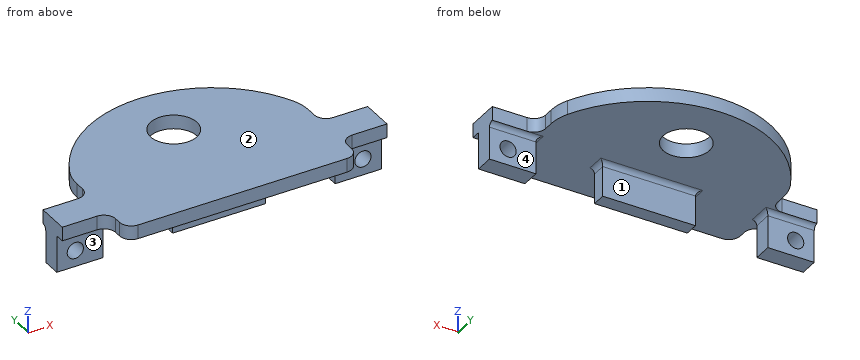
```python
from build123d import *

# Parameters (mm, degrees)
SKETCH1_W           = 20
SKETCH1_H           = 155
BOSS_EXTRUDE1_DEPTH = 4
SKETCH2_W           = 20
SKETCH2_H           = 4
BOSS_EXTRUDE3_DEPTH = 50
RIB2_REACH          = 96.986
SKETCH7_WALL_W      = 290.205463948
SKETCH7_WALL_H      = 4
SKETCH8_W           = 20
SKETCH8_H           = 3
BOSS_EXTRUDE4_DEPTH = 3.5
SKETCH9_W           = 70
SKETCH9_H           = 5
BOSS_EXTRUDE6_DEPTH = 3
SKETCH10_W          = 10
SKETCH10_H          = 4
BOSS_EXTRUDE7_DEPTH = 8
SKETCH12_R          = 1.75
CUT_EXTRUDE1_DEPTH  = 10
SKETCH13_W          = 111.319070758
SKETCH13_H          = 99.743885808
CUT_EXTRUDE2_DEPTH  = 152
SKETCH14_W          = 50
SKETCH14_H          = 3
BOSS_EXTRUDE8_DEPTH = 6.5
FILLET1_R           = 1
FILLET2_R           = 2.5
SKETCH15_R          = 5
BOSS_EXTRUDE9_DEPTH = 3
FILLET3_R           = 10


with BuildPart() as part:
    # Sketch1 → Boss-Extrude1 (new body)
    with BuildSketch(Plane.XY):
        Rectangle(SKETCH1_W, SKETCH1_H)
    extrude(amount=BOSS_EXTRUDE1_DEPTH)

    # Sketch2 → Boss-Extrude3 (add)
    with BuildSketch(Plane.XY.offset(4)):
        with Locations((0, -75.5)):
            Rectangle(SKETCH2_W, SKETCH2_H)
    extrude(amount=BOSS_EXTRUDE3_DEPTH)

    # Sketch7 wall → Rib2 (add, up to next)
    with BuildSketch(Plane(origin=(0, -26, 16.5), x_dir=(0, 0.967074537263, -0.25449329928), z_dir=(0, 0.25449329928, 0.967074537263)), mode=Mode.PRIVATE) as rib2_sk1:
        Rectangle(SKETCH7_WALL_W, SKETCH7_WALL_H)
    rib2_tool1 = extrude(rib2_sk1.sketch, amount=-RIB2_REACH, mode=Mode.PRIVATE) - part.part
    add(rib2_tool1.solids().sort_by_distance((0, -26, 16.5))[0])

    # Sketch8 → Boss-Extrude4 (add)
    with BuildSketch(Plane.XY.offset(4)):
        with Locations((0, 76)):
            Rectangle(SKETCH8_W, SKETCH8_H)
    extrude(amount=BOSS_EXTRUDE4_DEPTH)

    # Sketch9 → Boss-Extrude6 (add)
    with BuildSketch(Plane.XY.offset(7.5)):
        with Locations((0, 77)):
            Rectangle(SKETCH9_W, SKETCH9_H)
    boss_extrude6 = extrude(amount=BOSS_EXTRUDE6_DEPTH)

    # Sketch10 → Boss-Extrude7 (add)
    with BuildSketch(Plane(origin=(0, 0, 7.5), x_dir=(-1, 0, 0), z_dir=(0, 0, -1))):
        with Locations((30, 76.5)):
            Rectangle(SKETCH10_W, SKETCH10_H)
        with Locations((-30, 76.5)):
            Rectangle(SKETCH10_W, SKETCH10_H)
    extrude(amount=BOSS_EXTRUDE7_DEPTH)

    # Sketch12 → Cut-Extrude1 (cut)
    with BuildSketch(Plane(origin=(0, 78.5, 0), x_dir=(1, 0, 0), z_dir=(0, 1, 0))):
        with Locations(Location((-31, -3, 0), (0, 0, 270))):
            Circle(SKETCH12_R)
        with Locations(Location((31, -3, 0), (0, 0, 270))):
            Circle(SKETCH12_R)
    extrude(amount=-CUT_EXTRUDE1_DEPTH, mode=Mode.SUBTRACT)

    # Sketch13 → Cut-Extrude2 (cut)
    with BuildSketch(Plane.XZ.offset(77.5)):
        with Locations((2.652852139, 20.474703111)):
            Rectangle(SKETCH13_W, SKETCH13_H)
    extrude(amount=-CUT_EXTRUDE2_DEPTH, mode=Mode.SUBTRACT)

    # Sketch14 → Boss-Extrude8 (add)
    with BuildSketch(Plane(origin=(0, 79.5, 0), x_dir=(1, 0, 0), z_dir=(0, 1, 0))):
        with Locations((0, -9)):
            Rectangle(SKETCH14_W, SKETCH14_H)
    boss_extrude8 = extrude(amount=BOSS_EXTRUDE8_DEPTH)

    # Mirror1: Boss-Extrude6, Boss-Extrude8 across plane
    add(boss_extrude6.mirror(Plane(origin=(0, 76, 0), x_dir=(0, 0, 1), z_dir=(0, -1, 0))))
    add(boss_extrude8.mirror(Plane(origin=(0, 76, 0), x_dir=(0, 0, 1), z_dir=(0, -1, 0))))

    # Fillet1
    fillet1_edges = [part.edges().sort_by_distance(p)[0] for p in [
        (30, 78.5, 7.5),
        (-30, 78.5, 7.5),
        (10, 76, 7.5),
        (-10, 76, 7.5),
        (0, 77.5, 7.5),
        (25, 76.5, 7.5),
        (-25, 76.5, 7.5),
    ]]
    fillet(fillet1_edges, radius=FILLET1_R - 0.0001)  # a hair under: the kernel refuses the full size

    # Fillet2
    fillet2_edges = [part.edges().sort_by_distance(p)[0] for p in [
        (-25, 79.5, 9),
        (25, 79.5, 9),
        (-25, 66, 9),
        (25, 66, 9),
        (-25, 72.5, 9),
        (25, 72.5, 9),
    ]]
    fillet(fillet2_edges, radius=FILLET2_R)

    # Sketch15 → Boss-Extrude9 (add)
    with BuildSketch(Plane(origin=(0, 0, 7.5), x_dir=(-1, 0, 0), z_dir=(0, 0, -1))):
        with BuildLine():
            Line((25, 86), (-25, 86))
            ThreePointArc((-25, 86), (0, 103.502), (25, 86))
        make_face()
        with Locations((0, 91.001)):
            Circle(SKETCH15_R, mode=Mode.SUBTRACT)
    extrude(amount=-BOSS_EXTRUDE9_DEPTH)

    # Fillet3
    fillet3_edges = [part.edges().sort_by_distance(p)[0] for p in [
        (-25, 86, 9),
        (25, 86, 9),
    ]]
    fillet(fillet3_edges, radius=FILLET3_R)


solid = part.part
```
Here's how the part is built. I have some questions about the finished solid (model axes, mm). Face numbers are marked on the shaded views. A direction names the side the tool comes from. Give positions to 0.01 mm unless a question says otherwise; leave off trailing zeros. Loops run counter-clockwise (first coordinate to the right, second up) from the corner with the lowest first, then second, coordinate; pieces in that order, holes last. Notation, with made-up numbers: M 71.5,8.5 L 123.5,8.5 A15 ccw 123.5,34.5 Z; hole C 13,65.25 d2. An arc over 180 degrees is marked long. Return JSON: item names as keys, results as strings.
Item 1: Thinking about a two-plate mould opening in X: for the marked faces 1 and 2, which applies, released by +X, released by -X, zero draft, split by the parting line, or undercut?
A:
{"face 1": "undercut", "face 2": "zero draft"}
Item 2: On a 3-axis mill with a long thin cutter (end or side, diameter ignored), from which of +Z, -Z, +X, -X, +Y, -Y can I reach the whole of each face in a straight line? I mean the marked faces 3 and 4. Say none if no direction works.
A:
{"face 3": "-Z, +X, -X, -Y", "face 4": "-Z, +X, -X, +Y"}
Item 3: I'm going to push flat-ended pins straight in: pin 1 Ø4 at (x, z) = (27, 4.5) entering from -Y; pin 2 Ø4 at (x, y) = (10, 88.5) entering from -Z; pin 3 Ø0.9 at (x, z) = (-33, 9.5) entering from -Y; pin 4 Ø1 at (x, z) = (23, 3.5) entering from -Y. Where does each tip first touch, or does it pass through?
A:
{"pin 1": "stops at y = 74.5", "pin 2": "stops at z = 7.5", "pin 3": "stops at y = 72.5", "pin 4": "passes through"}
Item 4: Imagine slicing it at C-C on x = -26. List the corners of the cut face in (y, z) for me, then the cut area to 3 significant figures.
A:
{"outline": "M 72,7.5 L 74.5,7.5 L 74.5,-0.5 L 78.5,-0.5 L 78.5,6.5 A1 cw 79.5,7.5 L 80,7.5 L 80,10.5 L 72,10.5 Z", "area": "56.2 mm^2"}
Item 5: Imagine slicing it at B-B on z = 3. List the corners of the cut face in (x, y) for me, then the cut area to 3 significant figures.
A:
{"outline": "M -35,74.5 L -32.75,74.5 L -32.75,78.5 L -35,78.5 Z; M -29.25,74.5 L -25,74.5 L -25,78.5 L -29.25,78.5 Z; M -10,74.5 L 10,74.5 L 10,77.5 L -10,77.5 Z; M 25,74.5 L 29.25,74.5 L 29.25,78.5 L 25,78.5 Z; M 32.75,74.5 L 35,74.5 L 35,78.5 L 32.75,78.5 Z", "area": "112 mm^2"}
Item 6: Please list where these lines run through material, in increasing order: line 1 (X direction, y = 77.75, z = 3); line 2 (X direction, y = 75, z = 3.75); line 3 (X direction, y = 77.3, z = 3).
A:
{"line 1": "x = -35 to -32.75, -29.25 to -25, 25 to 29.25, 32.75 to 35", "line 2": "x = -35 to -32.58, -29.42 to -25, -10 to 10, 25 to 29.42, 32.58 to 35", "line 3": "x = -35 to -32.75, -29.25 to -25, -10 to 10, 25 to 29.25, 32.75 to 35"}
Item 7: Imagine slicing it at D-D on y = 94.5. List the corners of the cut face in (x, z) for me, then the cut area to 3 significant figures.
A:
{"outline": "M -19.95,7.5 L -3.57,7.5 L -3.57,10.5 L -19.95,10.5 Z; M 3.57,7.5 L 19.95,7.5 L 19.95,10.5 L 3.57,10.5 Z", "area": "98.3 mm^2"}
Item 8: Imagine slicing it at A-A on x = 0. List the corners of the cut face in (y, z) for me, then the cut area to 3 significant figures.
A:
{"outline": "M 66,7.5 L 74.5,7.5 L 74.5,0 L 77.5,0 L 77.5,6.5 A1 cw 78.5,7.5 L 86,7.5 L 86,10.5 L 66,10.5 Z; M 96,7.5 L 103.5,7.5 L 103.5,10.5 L 96,10.5 Z", "area": "105 mm^2"}
